CAD build for the part. Positions are in the model's coordinates, mm. A direction names the side the tool comes from. Give positions to 0.01 mm unless a question says otherwise; leave off trailing zeros. Loops run counter-clockwise (first coordinate to the right, second up) from the corner with the lowest first, then second, coordinate; pieces in that order, holes last.
Item 1: Saw through at B-B on y = 42.8. Give the cut face in (x, z).
Item 2: Probe probe 1 along Z at (x, y) = (-5.5, 1.4); probe 2 along Z at (x, y) = (-4, 43); probe 3 along Y at (x, z) = (-7.5, -15). List the from-to ranges inside material, lowest first.
Item 3: Which spindle directions (+Z, -Z, +X, -X, +Y, -Y) get a long thin tool onto all of the face, cutting with end or side? Do faces 4 (the flat face through (0, 3, -32.5)), 5 (the flat face through (-7, 27, 21)). Say none if no direction does.
Item 4: Mould opens along X. For faces 1 (the cylindrical face through (-5.796, 13.324, -14.868)), 2 (the cylindrical face through (7.206, 2.958, 28.808)), 3 (the flat face through (-2.5, 36, -9)) say: released by +X, released by -X, zero draft, split by the parting line, or undercut.
Item 5: Drop flat-ended pins along their axis: P1, Ø6.5, axis at x = -6.5, y = 21, coming from the -Z side; P2, Ø2.5, axis at x = -5.5, z = 27.5, coming from the +Y side; P3, Ø12, axis at x = 8.5, z = 8, coming from the +Y side; P4, Ø4, axis at y = 42.8, z = 15.5, coming from the +X side. Give the stop position or say it passes through.
Item 6: Saw through at A-A on x = -5.5. Give the cut face in (y, z).
Item 7: Saw through at D-D on z = 10. Give the cut face in (x, y).
Item 8: Saw through at C-C on z = 27.5. Give the cut face in (x, y).
Autodesk Inventor part; units mm, degrees
ref_plane "YZ Plane" through (0, 0, 0) normal (1, 0, 0) x (0, 1, 0)
ref_plane "XZ Plane" through (0, 0, 0) normal (0, 1, 0) x (-1, 0, 0)
ref_plane "XY Plane" through (0, 0, 0) normal (0, 0, 1) x (1, 0, 0)
sketch "Boceto1" plane through (0, 0, 0) normal (0, 1, 0) x (-1, 0, 0)
  line L0 (-10.5, 32.5) -> (10.5, 32.5)
  line L1 (10.5, 32.5) -> (10.5, -32.5)
  line L2 (10.5, -32.5) -> (-10.5, -32.5)
  line L3 (-10.5, -32.5) -> (-10.5, 32.5)
  line L4 (-10.5, 32.5) -> (10.5, -32.5) construction
  line L5 (10.5, 32.5) -> (-10.5, -32.5) construction
  circle A0 centre (5.5, 27.5) radius 2.15
  circle A1 centre (-5.5, 27.5) radius 2.15
  circle A2 centre (5.5, -27.5) radius 2.15
  circle A3 centre (-5.5, -27.5) radius 2.15
  point P0 (0, 0)
  dimension "d0" = 4.3
  dimension "d1" = 55
  dimension "d2" = 65
  dimension "d3" = 11
  dimension "d4" = 5
  dimension "d5" = 21
  dimension "d6" = 5
extrude "Extrusión1" add sketch "Boceto1" along normal blind 6
sketch "Boceto2" plane through (0, 6, 0) normal (0, 1, 0) x (1, 0, 0)
  line L0 (-10.5, 32.5) -> (-10.5, -32.5)
  line L1 (-10.5, -21) -> (-2.5, -21)
  line L2 (-2.5, -21) -> (-2.5, 21)
  line L3 (-2.5, 21) -> (-10.5, 21)
  line L4 (-10.5, 21) -> (-10.5, -21)
  point P0 (0, 0)
  point P1 (-10.5, 21)
  dimension "d9" = 42
  dimension "d10" = 21
  dimension "d11" = 8
extrude "Extrusión2" add sketch "Boceto2" along normal blind 42.3
sketch "Boceto3" plane through (-10.5, 0, -32.5) normal (-1, 0, 0) x (0, 0, 1)
  line L0 (11.5, 48.3) -> (53.5, 48.3)
  line L1 (53.5, 6) -> (53.5, 48.3)
  line L2 (11.5, 48.3) -> (53.5, 48.3)
  line L3 (53.5, 48.3) -> (53.5, 6.3)
  line L4 (53.5, 6.3) -> (11.5, 6.3)
  line L5 (11.5, 6.3) -> (11.5, 48.3)
  circle A0 centre (32.5, 27.3) radius 11.15
  point P0 (32.5, 0)
  dimension "d14" = 42
  dimension "d15" = 22.3
  dimension "d16" = 21
  dimension "d17" = 21
extrude "Extrusión3" cut sketch "Boceto3" against normal through all contours A0
sketch "Boceto4" plane through (-10.5, 0, -32.5) normal (-1, 0, 0) x (0, 0, 1)
  circle A0 centre (17, 42.8) radius 1.65
  circle A1 centre (32.5, 27.3) radius 11.15
  point P0 (32.5, 0)
  dimension "d20" = 15.5
  dimension "d22" = 15.5
  dimension "d23" = 3.3
extrude "Extrusión4" cut sketch "Boceto4" against normal through all contours A0
chamfer "Chaflán1" distance 1.5 angle 45 1 edges at (-10.5, 42.8, -17.15)
pattern_circular "Patrón circular1" count 4 over 360 about axis through (-10.5, 27.3, 0) along (1, 0, 0) of "Extrusión4", "Chaflán1"
properties part number "elbowmotorsupport"
Results below:
1. outline: (-10.5, -21) - (-2.5, -21) - (-2.5, -17.15) - (-9, -17.15) - (-10.5, -18.65) - close; (-10.5, -12.35) - (-9, -13.85) - (-2.5, -13.85) - (-2.5, 13.85) - (-9, 13.85) - (-10.5, 12.35) - close; (-10.5, 18.65) - (-9, 17.15) - (-2.5, 17.15) - (-2.5, 21) - (-10.5, 21) - close
2. probe 1: z = -32.5 to -29.65, -25.35 to 25.35, 29.65 to 32.5
2. probe 2: z = -21 to -17.14, -13.86 to 13.86, 17.14 to 21
2. probe 3: y = 0 to 10.23, 13.37 to 41.23, 44.37 to 48.3
3. face 4: -Z, +X, -X, +Y, -Y
3. face 5: +Z, +X, -X, +Y
4. face 1: zero draft
4. face 2: undercut
4. face 3: released by +X
5. P1: stops at z = -21
5. P2: passes through
5. P3: stops at y = 6
5. P4: stops at x = -2.5
6. outline: (0, -32.5) - (6, -32.5) - (6, -29.65) - (0, -29.65) - close; (0, -25.35) - (6, -25.35) - (6, -21) - (48.3, -21) - (48.3, 21) - (6, 21) - (6, 25.35) - (0, 25.35) - close; (0, 29.65) - (6, 29.65) - (6, 32.5) - (0, 32.5) - close; hole circle Ø3.3 at (11.8, -15.5); hole circle Ø3.3 at (11.8, 15.5); hole circle Ø22.3 at (27.3, 0); hole circle Ø3.3 at (42.8, -15.5); hole circle Ø3.3 at (42.8, 15.5)
7. outline: (-10.5, 0) - (10.5, 0) - (10.5, 6) - (-2.5, 6) - (-2.5, 22.37) - (-10.5, 22.37) - close; (-10.5, 32.23) - (-2.5, 32.23) - (-2.5, 48.3) - (-10.5, 48.3) - close
8. outline: (-10.5, 0) - (-7.65, 0) - (-7.65, 6) - (-10.5, 6) - close; (-3.35, 0) - (3.35, 0) - (3.35, 6) - (-3.35, 6) - close; (7.65, 0) - (10.5, 0) - (10.5, 6) - (7.65, 6) - close
